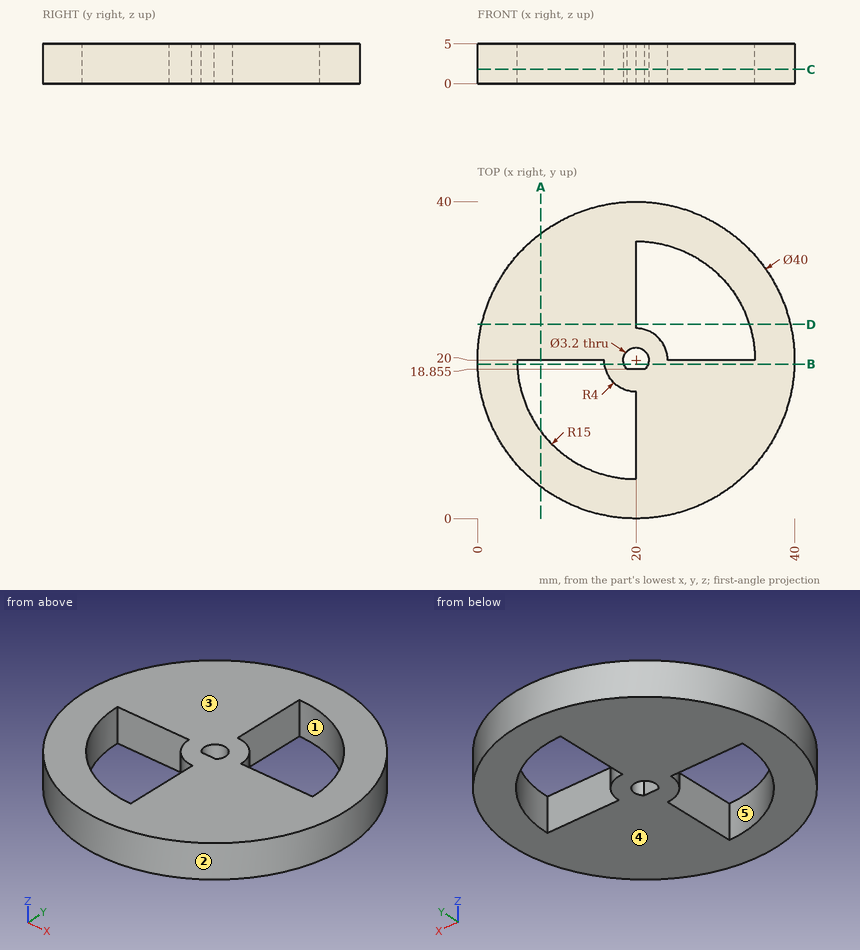
Input: dimensioned drawing with shaded views. Units: mm. Origin: part minimum x, y, z. A direction names the side the tool comes from. Coordinates: 2 decimals unless noted, no trailing zeros. Write each loop counter-clockwise with the first axis right and the second up, starting at its lowest first coordinate (ties: lowest second). Pieces come first, ordered by that corner, then holes. Notation, with made-up numbers: (16.5, 55) -> (58.5, 55) arc R14 ccw to (58.5, 72) -> close; hole circle Ø4 at (1, 59.5). An arc over 180 degrees is marked (long way). Return JSON: item names as keys, results as strings. Group by question number.
1) Contact query for flat-ended pins moving along their axis: P1, Ø1.8, axis at x = 19.5, z = 3.5, coming from the +Y side; P2, Ø1.5, axis at x = 30, z = 2, coming from the +Y side; P3, Ø12, axis at x = 31, y = 34, coming from the -Z side; P4, Ø1.5, axis at y = 17.5, z = 2, coming from the +X side. Output: stop coordinate, or through.
2) Section query D-D, the plane y = 24.5. Return loops of the section in (x, z), plus the area to 3 significant figures.
3) Section query A-A, the plane x = 8. Return loops of the section in (y, z).
4) Ray query, line 1 along X through (y, z) = (22, 1.3) (1 decimal); line 2 along X through (y, z) = (29, 1.35); line 3 along Y through (x, z) = (31, 2.4) (1 decimal). Return the intervals inside material, ascending.
5) Mould query, pull axis Y, two halves, no side actions, for the marked faces 1, 2 and 3. Classes: +Y half, -Y half, draft (parallel to the pull), parting line (faces both ways), or undercut.
6) Section query C-C, the plane z = 1.8. Return loops of the section in (x, y) (1 decimal), plus the area to 3 significant figures.
7) Section query B-B, the plane y = 19.5. Return loops of the section in (x, z).
8) Set-up query: the marked faces 4 and 5. Return all of +Z, -Z, +X, -X, +Y, -Y with unobstructed straight access to the full face (end or side cutting, diameter ignored); none if empty.
From the geometry:
{
 "1": {"P1": "y = 40", "P2": "y = 37.73", "P3": "z = 0", "P4": "x = 39.92"},
 "2": {"outline": "(0.51, 0) -> (20, 0) -> (20, 5) -> (0.51, 5) -> close; (34.31, 0) -> (39.49, 0) -> (39.49, 5) -> (34.31, 5) -> close", "area": "123 mm²"},
 "3": {"outline": "(4, 0) -> (11, 0) -> (11, 5) -> (4, 5) -> close; (20, 0) -> (36, 0) -> (36, 5) -> (20, 5) -> close"},
 "4": {"line 1": "0.1 to 23.5, 34.9 to 39.9", "line 2": "2.14 to 20, 32 to 37.86", "line 3": "3.3 to 20, 30.2 to 36.7"},
 "5": {"face 1": "undercut", "face 2": "parting line", "face 3": "draft"},
 "6": {"outline": "circle Ø40 at (20, 20); hole (5, 20) arc R15 ccw to (20, 5) -> (20, 16) arc R4 cw to (16, 20) -> close; hole (18.9, 18.9) -> (21.1, 18.9) arc R1.6 ccw (long way) to start; hole (20, 24) arc R4 cw to (24, 20) -> (35, 20) arc R15 ccw to (20, 35) -> close", "area": "921 mm²"},
 "7": {"outline": "(0.01, 0) -> (5.01, 0) -> (5.01, 5) -> (0.01, 5) -> close; (16.03, 0) -> (18.48, 0) -> (18.48, 5) -> (16.03, 5) -> close; (21.52, 0) -> (39.99, 0) -> (39.99, 5) -> (21.52, 5) -> close"},
 "8": {"face 4": "-Z, +X, -X, +Y, -Y", "face 5": "+Z, -Z"}
}
